Work out the finished part from the listing and answer in its coordinate system (mm). Coordinates: 2 decimals unless noted, no trailing zeros. Write each loop counter-clockwise with the first axis right and the second up, starting at its lowest first coordinate (ties: lowest second). Pieces come first, ordered by that corner, then holes. Notation, with made-up numbers: (15.5, 12.25) - (54.5, 12.25) arc R25 cw to (54.5, 35.25) - close; hole circle Ø4 at (-23, 0). An arc over 180 degrees is marked (long way). Use a Markdown table: item, result. Add a question column.
(1) Find the intervals of material crossed by line 1 (Z direction, x = 318.5, y = 1532.5); line 2 (Z direction, x = 898.5, y = 1535.25); line 3 (Z direction, x = 737.5, y = 1535.5), in increasing order. Write a range as from..to.
(2) The part is cut by section A-A, the plane z = 1746. Give the vertices of the cut face in (x, y).
(3) The part is cut by section D-D, the plane x = 607. Give the vertices of the cut face in (y, z).
(4) The part is cut by section C-C, the plane y = 1531.75. Give the vertices of the cut face in (x, z), then the cut area to 3 significant figures.
(5) The part is cut by section B-B, the plane x = 769.5. Give the vertices of the cut face in (y, z).
from build123d import *

# Parameters (mm, degrees)
SKETCH023_W            = 1422.4
SKETCH023_H            = 1625.6
SKETCH023_W_2          = 406.4
SKETCH023_H_2          = 457.2
SKETCH023_W_3          = 914.4
PAD004_DEPTH           = 12.7
SKETCH024_W            = 203.2
SKETCH024_H            = 127
POCKET019_DEPTH        = 12.7010000028
LINEARPATTERN001_COUNT = 4
LINEARPATTERN001_PITCH = 338.6666666667


with BuildPart() as part:
    # Sketch023 → Pad004 (new body)
    with BuildSketch(Plane(origin=(0, 1524, 0), x_dir=(1, 0, 0), z_dir=(0, -1, 0))):
        with Locations((762, 1358.9)):
            Rectangle(SKETCH023_W, SKETCH023_H)
        with Locations((762, 1041.4)):
            Rectangle(SKETCH023_W_2, SKETCH023_H_2, mode=Mode.SUBTRACT)
        with Locations((728.768672, 1716.358264)):
            Rectangle(SKETCH023_W_3, SKETCH023_H_2, mode=Mode.SUBTRACT)
    extrude(amount=-PAD004_DEPTH)

    # Sketch024 → Pocket019 (cut, through all)
    with BuildSketch(Plane(origin=(0, 1536.7, 0), x_dir=(1, 0, 0), z_dir=(0, 1, 0))):
        with Locations((254, -2057.4)):
            Rectangle(SKETCH024_W, SKETCH024_H)
    pocket019 = extrude(amount=-POCKET019_DEPTH, mode=Mode.SUBTRACT)

    # LinearPattern001: Pocket019 ×4
    with Locations(*[(i * LINEARPATTERN001_PITCH, 0, 0) for i in range(1, LINEARPATTERN001_COUNT)]):
        add(pocket019, mode=Mode.SUBTRACT)


solid = part.part
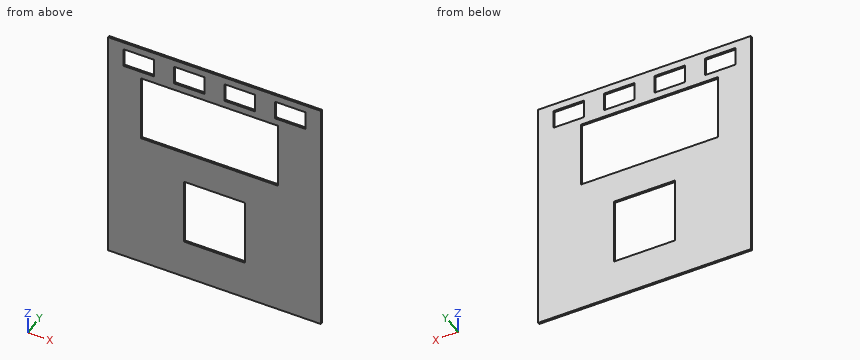
Model answer:
| question | item | result |
|---|---|---|
| 1 | line 1 | 546.1..1487.76, 1944.96..1993.9, 2120.9..2171.7 |
| 1 | line 2 | 546.1..812.8, 1270..1487.76, 1944.96..1993.9, 2120.9..2171.7 |
| 1 | line 3 | 546.1..812.8, 1270..1487.76, 1944.96..2171.7 |
| 2 | outline | (50.8, 1524) - (271.57, 1524) - (271.57, 1536.7) - (50.8, 1536.7) - close; (1185.97, 1524) - (1473.2, 1524) - (1473.2, 1536.7) - (1185.97, 1536.7) - close |
| 3 | outline | (1524, 546.1) - (1536.7, 546.1) - (1536.7, 812.8) - (1524, 812.8) - close; (1524, 1270) - (1536.7, 1270) - (1536.7, 1487.76) - (1524, 1487.76) - close; (1524, 1944.96) - (1536.7, 1944.96) - (1536.7, 1993.9) - (1524, 1993.9) - close; (1524, 2120.9) - (1536.7, 2120.9) - (1536.7, 2171.7) - (1524, 2171.7) - close |
| 4 | outline | (50.8, 546.1) - (1473.2, 546.1) - (1473.2, 2171.7) - (50.8, 2171.7) - close; hole (152.4, 1993.9) - (355.6, 1993.9) - (355.6, 2120.9) - (152.4, 2120.9) - close; hole (271.57, 1487.76) - (1185.97, 1487.76) - (1185.97, 1944.96) - (271.57, 1944.96) - close; hole (491.07, 1993.9) - (694.27, 1993.9) - (694.27, 2120.9) - (491.07, 2120.9) - close; hole (558.8, 812.8) - (965.2, 812.8) - (965.2, 1270) - (558.8, 1270) - close; hole (829.73, 1993.9) - (1032.93, 1993.9) - (1032.93, 2120.9) - (829.73, 2120.9) - close; hole (1168.4, 1993.9) - (1371.6, 1993.9) - (1371.6, 2120.9) - (1168.4, 2120.9) - close |
| 4 | area | 1,610,000 mm^2 |
| 5 | outline | (1524, 546.1) - (1536.7, 546.1) - (1536.7, 812.8) - (1524, 812.8) - close; (1524, 1270) - (1536.7, 1270) - (1536.7, 1487.76) - (1524, 1487.76) - close; (1524, 1944.96) - (1536.7, 1944.96) - (1536.7, 2171.7) - (1524, 2171.7) - close |
